The model under review builds one solid part; all positions refer to its coordinate system, in mm. A direction names the side the tool comes from. Give positions to 0.01 mm unless a question says otherwise; leave off trailing zeros. Order: outer loops, then holes, each group sorted by start corner. A loop starts at its lowest first (then second) coordinate and runs counter-clockwise, first axis right, second up.
```python
from build123d import *

# Parameters (mm, degrees)
BOSS_EXTRUDE1_DEPTH = 20
FILLET1_R           = 3
CUT_EXTRUDE1_REACH  = 51.8
SKETCH3_R           = 1.6
CUT_EXTRUDE2_REACH  = 51.8
SKETCH4_R           = 1.25


with BuildPart() as part:
    # Sketch1 → Boss-Extrude1 (new body)
    with BuildSketch(Plane(origin=(0, 0, 0), x_dir=(1, 0, 0), z_dir=(0, 1, 0))):
        Polygon((28, 12.528445914), (-28, 12.528445914), (-28, -10.471554086), (-36, -10.471554086), (-36, -15.471554086), (-23, -15.471554086), (-23, 7.528445914), (23, 7.528445914), (23, -15.471554086), (36, -15.471554086), (36, -10.471554086), (28, -10.471554086), align=None)
    extrude(amount=BOSS_EXTRUDE1_DEPTH)

    # Fillet1
    fillet1_edges = [part.edges().sort_by_distance(p)[0] for p in [
        (23, 10, -7.528445914),
        (-23, 10, -7.528445914),
    ]]
    fillet(fillet1_edges, radius=FILLET1_R)

    # Sketch3 → Cut-Extrude1 (cut, up to next)
    with BuildSketch(Plane.XY.offset(15.471554086), mode=Mode.PRIVATE) as cut_extrude1_sk1:
        with Locations((-32, 10)):
            Circle(SKETCH3_R)
    cut_extrude1_tool1 = extrude(cut_extrude1_sk1.sketch, amount=-CUT_EXTRUDE1_REACH, mode=Mode.PRIVATE) & part.part
    # Sketch3 → Cut-Extrude1 (cut, up to next)
    with BuildSketch(Plane.XY.offset(15.471554086), mode=Mode.PRIVATE) as cut_extrude1_sk2:
        with Locations((32, 10)):
            Circle(SKETCH3_R)
    cut_extrude1_tool2 = extrude(cut_extrude1_sk2.sketch, amount=-CUT_EXTRUDE1_REACH, mode=Mode.PRIVATE) & part.part
    add(cut_extrude1_tool1.solids().sort_by_distance((-32, 10, 15.471554))[0], mode=Mode.SUBTRACT)
    add(cut_extrude1_tool2.solids().sort_by_distance((32, 10, 15.471554))[0], mode=Mode.SUBTRACT)

    # Sketch4 → Cut-Extrude2 (cut, up to next)
    with BuildSketch(Plane(origin=(0, 0, -12.528445914), x_dir=(-1, 0, 0), z_dir=(0, 0, -1)), mode=Mode.PRIVATE) as cut_extrude2_sk1:
        with Locations((0, 10)):
            Circle(SKETCH4_R)
    cut_extrude2_tool1 = extrude(cut_extrude2_sk1.sketch, amount=-CUT_EXTRUDE2_REACH, mode=Mode.PRIVATE) & part.part
    add(cut_extrude2_tool1.solids().sort_by_distance((0, 10, -12.528446))[0], mode=Mode.SUBTRACT)


solid = part.part
```
Item 1: Draft analysis for pull direction Y (two halves, no side actions). For faces 1 (the flat face through (-1, 0, -8)), 2 (the cylindrical face through (-33.6, 10.07, 13.01)), 3 (the cylindrical face through (0.16, 11.24, -10.06)), 4 (the flat face through (-34, 10, 10.472)), state which applies: released by +Y, released by -Y, zero draft, split by the parting line, or undercut.
Values found:
face 1: released by -Y
face 2: undercut
face 3: undercut
face 4: zero draft
Item 2: Take a section at D-D (z = -1.5). Give the boundary of the cut face in (x, y).
Values found:
outline: (-28, 0) - (-23, 0) - (-23, 20) - (-28, 20) - close; (23, 0) - (28, 0) - (28, 20) - (23, 20) - close
Item 3: Take a section at C-C (y = 10). Give the boundary of the cut face in (x, z).
Values found:
outline: (-36, 10.47) - (-33.6, 10.47) - (-33.6, 15.47) - (-36, 15.47) - close; (-30.4, 10.47) - (-28, 10.47) - (-28, -12.53) - (-1.25, -12.53) - (-1.25, -7.53) - (-20, -7.53) arc R3 cw to (-23, -4.53) - (-23, 15.47) - (-30.4, 15.47) - close; (1.25, -12.53) - (28, -12.53) - (28, 10.47) - (30.4, 10.47) - (30.4, 15.47) - (23, 15.47) - (23, -4.53) arc R3 cw to (20, -7.53) - (1.25, -7.53) - close; (33.6, 10.47) - (36, 10.47) - (36, 15.47) - (33.6, 15.47) - close
Item 4: Take a section at A-A (z = 12.25). Give the boundary of the cut face in (x, y), and give its area (3 significant figures).
Values found:
outline: (-36, 0) - (-23, 0) - (-23, 20) - (-36, 20) - close; (23, 0) - (36, 0) - (36, 20) - (23, 20) - close; hole circle Ø3.2 at (-32, 10); hole circle Ø3.2 at (32, 10)
area: 504 mm2
Item 5: Clearance check with flat-ended pins moving along their axes: pin 1 Ø3 at (y, z) = (11.5, 7) entering from -X; pin 2 Ø6 at (x, y) = (-2, 8.5) entering from +Z; pin 3 Ø6.5 at (x, y) = (-33.5, 9) entering from -Z. State where each tip first meets the part, or that it passes through.
Values found:
pin 1: stops at x = -28
pin 2: stops at z = -7.53
pin 3: stops at z = 10.47
Item 6: For line 1 (Y direction, x = 0, z = -9.9); line 2 (X direction, y = 8.5, z = 8.75); line 3 (X direction, y = 17.5, z = 13), list the stretches that pass through material, from the lowest coordinate up.
Values found:
line 1: y = 0 to 8.75, 11.25 to 20
line 2: x = -28 to -23, 23 to 28
line 3: x = -36 to -23, 23 to 36
Item 7: Take a section at B-B (x = 0). Give the boundary of the cut face in (y, z), and give its area (3 significant figures).
Values found:
outline: (0, -12.53) - (8.75, -12.53) - (8.75, -7.53) - (0, -7.53) - close; (11.25, -12.53) - (20, -12.53) - (20, -7.53) - (11.25, -7.53) - close
area: 87.5 mm2
Item 8: For faces 5 (the flat face through (34, 10, 10.472)), 6 (the flat face through (36, 10, 13)), 7 (the cylindrical face through (-22.14, 10.14, -6.63)), 8 (the flat face through (-28, 10, -1)), list the 3-axis set-ups (+Z, -Z, +X, -X, +Y, -Y) from which the entire face can be reached by the end or side of a thin tool; tool diameter is ignored.
Values found:
face 5: -Z, +X, +Y, -Y
face 6: +Z, -Z, +X, +Y, -Y
face 7: +Z, +Y, -Y
face 8: -Z, -X, +Y, -Y
